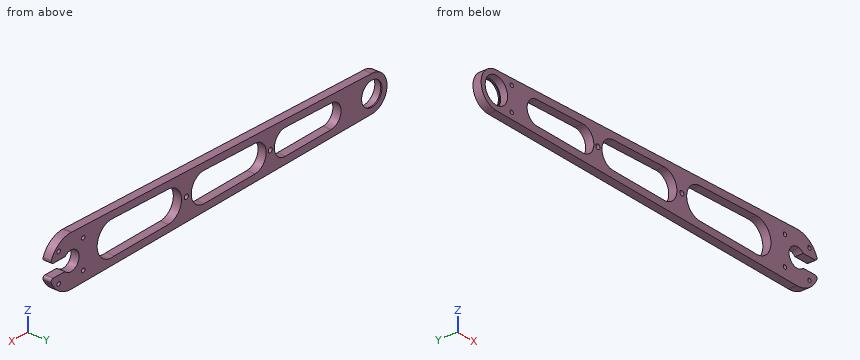
```python
from build123d import *

# Parameters (mm, degrees)
SKETCH1_R             = 10
BOSS_EXTRUDE1_DEPTH   = 7
CIRPATTERN1_COUNT     = 4
SKETCH4_R             = 11
CUT_EXTRUDE2_DEPTH    = 6
M4_TAPPED_HOLE1_D     = 3.3
M4_TAPPED_HOLE1_DEPTH = 5
M4_TAPPED_HOLE1_TIP   = 0.991420021
SKETCH7_R             = 2
CUT_EXTRUDE3_DEPTH    = 7


with BuildPart() as part:
    # Sketch1 → Boss-Extrude1 (new body)
    with BuildSketch(Plane(origin=(0, 0, 0), x_dir=(1, 0, 0), z_dir=(0, 1, 0))):
        with BuildLine():
            Line((246.627930173, -20.982691565), (247.480370611, -21))
            ThreePointArc((247.480370611, -21), (259.0328823, -17.536803406), (266.775049308, -8.289473684))
            ThreePointArc((266.775049308, -8.289473684), (266.607632614, -6.399760792), (264.937460861, -5.5))
            Line((264.937460861, -5.5), (253.28984563, -5.5))
            ThreePointArc((253.28984563, -5.5), (239.480370611, 0), (253.28984563, 5.5))
            Line((253.28984563, 5.5), (264.937460861, 5.5))
            ThreePointArc((264.937460861, 5.5), (266.607632614, 6.399760792), (266.775049308, 8.289473684))
            ThreePointArc((266.775049308, 8.289473684), (259.0328823, 17.536803406), (247.480370611, 21))
            Line((247.480370611, 21), (246.627930173, 20.982691565))
            Line((246.627930173, 20.982691565), (-48.019629389, 15))
            ThreePointArc((-48.019629389, 15), (-63.019629389, 0), (-48.019629389, -15))
            Line((-48.019629389, -15), (246.627930173, -20.982691565))
        make_face()
        with Locations(Location((-48.019629389, 0, 0), (0, 0, 270))):
            Circle(SKETCH1_R, mode=Mode.SUBTRACT)
    extrude(amount=BOSS_EXTRUDE1_DEPTH)

    # Sketch3 → Tap Drill for M4 Tap1 (revolve, cut)
    with BuildSketch(Plane(origin=(259.501185891, 7, -12.02081528), x_dir=(0, 0, 1), z_dir=(1, 0, 0))):
        Polygon((0, 0), (0, 8.991420021), (1.65, 8), (1.65, 0), align=None)
    tap_drill_for_m4_tap1 = revolve(axis=Axis((259.501185891, 13.35, -12.02081528), (0, -1, 0)), mode=Mode.SUBTRACT)

    # CirPattern1: Tap Drill for M4 Tap1 ×4 about axis
    cirpattern1_axis = Axis((247.480370611, 0, 0), (0, 1, 0))
    for i in range(1, CIRPATTERN1_COUNT):
        add(tap_drill_for_m4_tap1.rotate(cirpattern1_axis, i * 360 / CIRPATTERN1_COUNT), mode=Mode.SUBTRACT)

    # Sketch4 → Cut-Extrude2 (cut)
    with BuildSketch(Plane(origin=(0, 0, 0), x_dir=(1, 0, 0), z_dir=(0, 1, 0))):
        with Locations(Location((-48.019629389, 0, 0), (0, 0, 270))):
            Circle(SKETCH4_R)
    extrude(amount=CUT_EXTRUDE2_DEPTH, mode=Mode.SUBTRACT)

    # M4 Tapped Hole1
    with Locations(Plane(origin=(0, 0, 0), x_dir=(-1, 0, 0), z_dir=(0, -1, 0))):
        with Locations((33.019629389, -10), (33.019629389, 10)):
            Hole(M4_TAPPED_HOLE1_D / 2, depth=M4_TAPPED_HOLE1_DEPTH)
            with Locations((0, 0, -(M4_TAPPED_HOLE1_DEPTH + M4_TAPPED_HOLE1_TIP / 2))):  # 118° drill point
                Cone(0, M4_TAPPED_HOLE1_D / 2, M4_TAPPED_HOLE1_TIP, mode=Mode.SUBTRACT)

    # Sketch7 → Cut-Extrude3 (cut)
    with BuildSketch(Plane(origin=(0, 0, 0), x_dir=(-1, 0, 0), z_dir=(0, -1, 0))):
        with Locations(Location((-134.125113886, 0, 0), (0, 0, 90))):
            Circle(SKETCH7_R)
        with Locations(Location((-51.675864847, 0, 0), (0, 0, 90))):
            Circle(SKETCH7_R)
        with BuildLine():
            Line((8.218754321, -9.806902896), (-36.762700927, -10.720231937))
            ThreePointArc((-36.762700927, -10.720231937), (-47.702812165, 0), (-36.762700927, 10.720231937))
            Line((-36.762700927, 10.720231937), (8.218754321, 9.806902896))
            ThreePointArc((8.218754321, 9.806902896), (17.82855365, 0), (8.218754321, -9.806902896))
        make_face()
        with BuildLine():
            Line((-66.750337759, 11.329117964), (-116.729732479, 12.343928009))
            ThreePointArc((-116.729732479, 12.343928009), (-129.326842907, 0), (-116.729732479, -12.343928009))
            Line((-116.729732479, -12.343928009), (-66.750337759, -11.329117964))
            ThreePointArc((-66.750337759, -11.329117964), (-55.648917529, 0), (-66.750337759, 11.329117964))
        make_face()
        with BuildLine():
            Line((-151.715308783, -13.05429504), (-207.190686799, -14.180698655))
            ThreePointArc((-207.190686799, -14.180698655), (-221.709735655, 1.233303858), (-204.918313244, 14.13455909))
            Line((-204.918313244, 14.13455909), (-151.715308783, 13.05429504))
            ThreePointArc((-151.715308783, 13.05429504), (-138.923384865, 0), (-151.715308783, -13.05429504))
        make_face()
    extrude(amount=-CUT_EXTRUDE3_DEPTH, mode=Mode.SUBTRACT)


solid = part.part
```
Build history of the part. All positions in model axes, mm. Round coordinates to 2 decimals unless told otherwise and drop trailing zeros. Write each loop counter-clockwise with the first axis right and the second up, starting at its lowest first coordinate (ties: lowest second). Pieces come first, ordered by that corner, then holes. Notation, with made-up numbers: (-32.75, -28) - (21.25, -28) arc R22 ccw to (21.25, -6) - close; hole circle Ø9 at (-9.75, 11). An arc over 180 degrees is marked (long way). Write each question's results on one line, items separated by ' | '. Start each with the question number.
Item 1: Saw through at B-B (y = 1.25). State how many separate pieces and enclosed holes the cut face has, and give its area (3 significant figures).
Item 2: Saw through at A-A (x = 91). Write the cut outline in (y, z).
Item 3: Drop flat-ended pins along their axis: P1, Ø11, axis at x = -49, z = -2.5, coming from the -Y side; P2, Ø4, axis at x = 259.5, z = -12.02, coming from the +Y side; P3, Ø3.5, axis at x = 259.5, y = 4.5, coming from the +Z side; P4, Ø1.5, axis at x = 22, y = 3.5, coming from the +Z side. Give the stop position or say it passes through.
Item 4: Wall check: L1, parallel to X at y = 3.5, z = 3; L2, parallel to X at y = 5.5, z = 5; L3, parallel to Z at x = -11, y = 3.75. Give the ranges that are in metal, low to high. Write a range as [from, to].
Results are:
1) separate pieces: 1 | enclosed holes: 12 | area: 5,890 mm²
2) outline: (0, -17.82) - (7, -17.82) - (7, -11.82) - (0, -11.82) - close; (0, 11.82) - (7, 11.82) - (7, 17.82) - (0, 17.82) - close
3) P1: passes through | P2: stops at y = 7 | P3: stops at z = 18.32 | P4: stops at z = 16.44
4) L1: x = [-62.72, -58.6], [-37.44, -17.36], [47.27, 56.05], [128.96, 139.27], [221.42, 240.06] | L2: x = [-62.16, -57.82], [-38.22, -16.46], [46.47, 56.81], [128.27, 139.92], [220.82, 241.24] | L3: z = [-15.75, -9.35], [9.35, 15.75]
